from build123d import *

# Parameters (mm, degrees)
SCHIZZO1_W                = 88
SCHIZZO1_H                = 138
ESTRUSIONE_SOTTILE1_DEPTH = 1000
ESTRUSIONE1_DEPTH         = 1017.120071645
ESTRUSIONE2_DEPTH         = 1017.120071645
SCHIZZO4_R                = 30
ESTRUSIONE3_DEPTH         = 1017.120071645
SCHIZZO7_W                = 100
SCHIZZO7_H                = 360
ESTRUSIONE6_DEPTH         = 5
SCHIZZO6_R                = 6.5
ESTRUSIONE5_DEPTH         = 1017.870198206
ESTRUSIONE7_DEPTH         = 40
ESTRUSIONE7_DEPTH_BACK    = 40


with BuildPart() as part:
    # Schizzo1 → Estrusione-Sottile1 (new body)
    with BuildSketch(Plane.XY):
        with BuildLine():
            Line((5, 0), (95, 0))
            ThreePointArc((95, 0), (98.535533906, 1.464466094), (100, 5))
            Line((100, 5), (100, 145))
            ThreePointArc((100, 145), (98.535533906, 148.535533906), (95, 150))
            Line((95, 150), (5, 150))
            ThreePointArc((5, 150), (1.464466094, 148.535533906), (0, 145))
            Line((0, 145), (0, 5))
            ThreePointArc((0, 5), (1.464466094, 1.464466094), (5, 0))
        make_face()
        with Locations((50, 75)):
            Rectangle(SCHIZZO1_W, SCHIZZO1_H, mode=Mode.SUBTRACT)
    extrude(amount=ESTRUSIONE_SOTTILE1_DEPTH)

    # Schizzo2 → Estrusione1 (cut, through all)
    with BuildSketch(Plane(origin=(100, 0, 0), x_dir=(0, 0, -1), z_dir=(1, 0, 0))):
        Polygon((-920, 0), (-1000, 150), (-1000, 0), align=None)
    extrude(amount=-ESTRUSIONE1_DEPTH, mode=Mode.SUBTRACT)

    # Schizzo3 → Estrusione2 (cut, through all)
    with BuildSketch(Plane(origin=(100, 0, 0), x_dir=(0, 0, -1), z_dir=(1, 0, 0))):
        Polygon((-180, 150), (-260, 0), (0, 0), (0, 150), align=None)
    extrude(amount=-ESTRUSIONE2_DEPTH, mode=Mode.SUBTRACT)

    # Schizzo4 → Estrusione3 (cut, through all)
    with BuildSketch(Plane.XZ):
        with Locations(Location((50, 850, 0), (0, 0, 270))):
            Circle(SCHIZZO4_R)
    extrude(amount=-ESTRUSIONE3_DEPTH, mode=Mode.SUBTRACT)

    # Schizzo7 → Estrusione6 (add)
    with BuildSketch(Plane(origin=(0, 150, 0), x_dir=(1, 0, 0), z_dir=(0, 1, 0))):
        with Locations((50, -600)):
            Rectangle(SCHIZZO7_W, SCHIZZO7_H)
    extrude(amount=ESTRUSIONE6_DEPTH)

    # Schizzo6 → Estrusione5 (cut, through all)
    with BuildSketch(Plane.XZ):
        with Locations(Location((14, 725, 0), (0, 0, 270))):
            Circle(SCHIZZO6_R)
        with Locations(Location((14, 495, 0), (0, 0, 270))):
            Circle(SCHIZZO6_R)
        with Locations(Location((86, 495, 0), (0, 0, 270))):
            Circle(SCHIZZO6_R)
        with Locations(Location((86, 725, 0), (0, 0, 270))):
            Circle(SCHIZZO6_R)
    extrude(amount=-ESTRUSIONE5_DEPTH, mode=Mode.SUBTRACT)

    # Schizzo9 → Estrusione7 (add, two sides: drawn at the far end of the back side and taken through both)
    with BuildSketch(Plane.XY.offset(850).offset(-ESTRUSIONE7_DEPTH_BACK)):
        with BuildLine():
            Line((100, 60), (100, -40))
            Line((100, -40), (132, -40))
            Line((132, -40), (132, -37))
            ThreePointArc((132, -37), (131.121320344, -34.878679656), (129, -34))
            Line((129, -34), (111, -34))
            ThreePointArc((111, -34), (107.464466094, -32.535533906), (106, -29))
            Line((106, -29), (106, 57))
            ThreePointArc((106, 57), (105.121320344, 59.121320344), (103, 60))
            Line((103, 60), (100, 60))
        make_face()
    extrude(amount=ESTRUSIONE7_DEPTH + ESTRUSIONE7_DEPTH_BACK)


solid = part.part
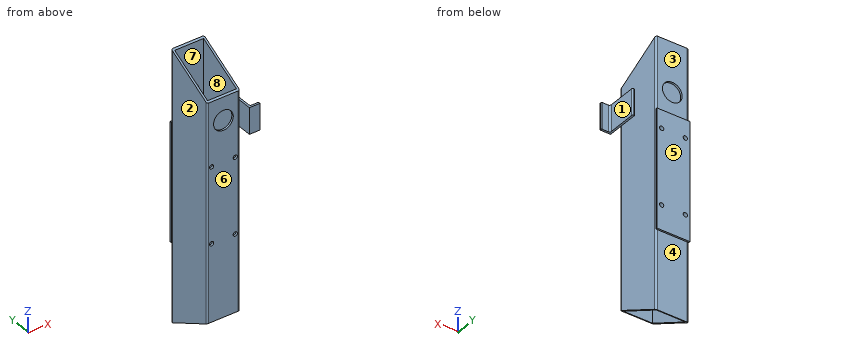
Build history of the part. All positions in model axes, mm. Face numbers are marked on the shaded views. A direction names the side the tool comes from. Coordinates: 2 decimals unless noted, no trailing zeros. Order: outer loops, then holes, each group sorted by start corner. A loop starts at its lowest first (then second) coordinate and runs counter-clockwise, first axis right, second up. Notation, with made-up numbers: (77.25, -38.75) - (94.25, -38.75) arc R27 cw to (94.25, -15.75) - close; hole circle Ø6 at (60.5, 32.5). An arc over 180 degrees is marked (long way). Write each question's results on one line, items separated by ' | '. Start each with the question number.
Item 1: Tool access for the marked faces 1, 2, 3 and 4: list every direction of +Z, -Z, +X, -X, +Y, -Y with a clear straight run to the whole face (end or side of a thin tool).
Item 2: Band-saw the part on A-A on y = 69. Write the cut outline in (x, z), and give its area (3 significant figures).
Item 3: Band-saw the part on B-B on x = 50. Write the cut outline in (y, z).
Item 4: Flat gauge pins, fed straight in: pin 1 (8 mm diameter, centred on y = 7.5, z = 671, fed in from +X); pin 2 (1.5 mm diameter, centred on x = 98, z = 592.5, fed in from -Y); pin 3 (20 mm diameter, centred on x = 121.5, z = 859.5, fed in from +Y). Where does each tip first touch, or does it go through?
Item 5: Wall check: probe 1 along X at (y, z) = (4, 495); probe 2 along X at (y, z) = (152.5, 495); probe 3 along X at (y, z) = (146, 850). Give the ranges that are in metal, low to high. Write a range as [from, to].
Item 6: Band-saw the part on D-D on z = 567.5. Write the cut outline in (x, y), and give its area (3 significant figures).
Item 7: Mould opens along Y. For the marked faces 5, 6, 7 and 8 say: released by +Y, released by -Y, zero draft, split by the parting line, or undercut.
Numbers:
1) face 1: +Z, -Z, +X, +Y | face 2: +Z, -Z, -X, +Y, -Y | face 3: +Z, +X, -X, +Y | face 4: -Z, +X, -X, +Y
2) outline: (0, 223.2) - (6, 223.2) - (6, 956.8) - (0, 956.8) - close; (94, 223.2) - (100, 223.2) - (100, 956.8) - (94, 956.8) - close | area: 8,800 mm^2
3) outline: (0, 260) - (6, 256.8) - (6, 820) - (0, 820) - close; (0, 880) - (6, 880) - (6, 923.2) - (0, 920) - close; (144, 183.2) - (150, 180) - (150, 420) - (155, 420) - (155, 780) - (150, 780) - (150, 820) - (144, 820) - close; (144, 880) - (150, 880) - (150, 1000) - (144, 996.8) - close
4) pin 1: x = 100 | pin 2: y = 0.53 | pin 3: y = -34
5) probe 1: [0.1, 7.5], [20.5, 79.5], [92.5, 99.9] | probe 2: [0, 7.5], [20.5, 79.5], [92.5, 100] | probe 3: [0.1, 20], [80, 99.9]
6) outline: (0, 5) arc R5 ccw to (5, 0) - (95, 0) arc R5 ccw to (100, 5) - (100, 145) arc R5 ccw to (95, 150) - (100, 150) - (100, 155) - (0, 155) - (0, 150) - (5, 150) arc R5 ccw to (0, 145) - close; hole (6, 6) - (94, 6) - (94, 144) - (6, 144) - close | area: 3,330 mm^2
7) face 5: released by +Y | face 6: released by -Y | face 7: undercut | face 8: undercut
